The drawing under review shows one solid part. Ordinate dimensions are in mm from its lowest x, y, z. Coordinates: 2 decimals unless noted, no trailing zeros. Order: outer loops, then holes, each group sorted by start corner. A loop starts at its lowest first (then second) coordinate and runs counter-clockwise, first axis right, second up. Notation, with made-up numbers: (-33, 43) - (-11, 43) arc R35 ccw to (-11, 78) - close; hole circle Ø10 at (-13, 45.25). An arc over 180 degrees is marked (long way). Answer in a Markdown table with one row per item.
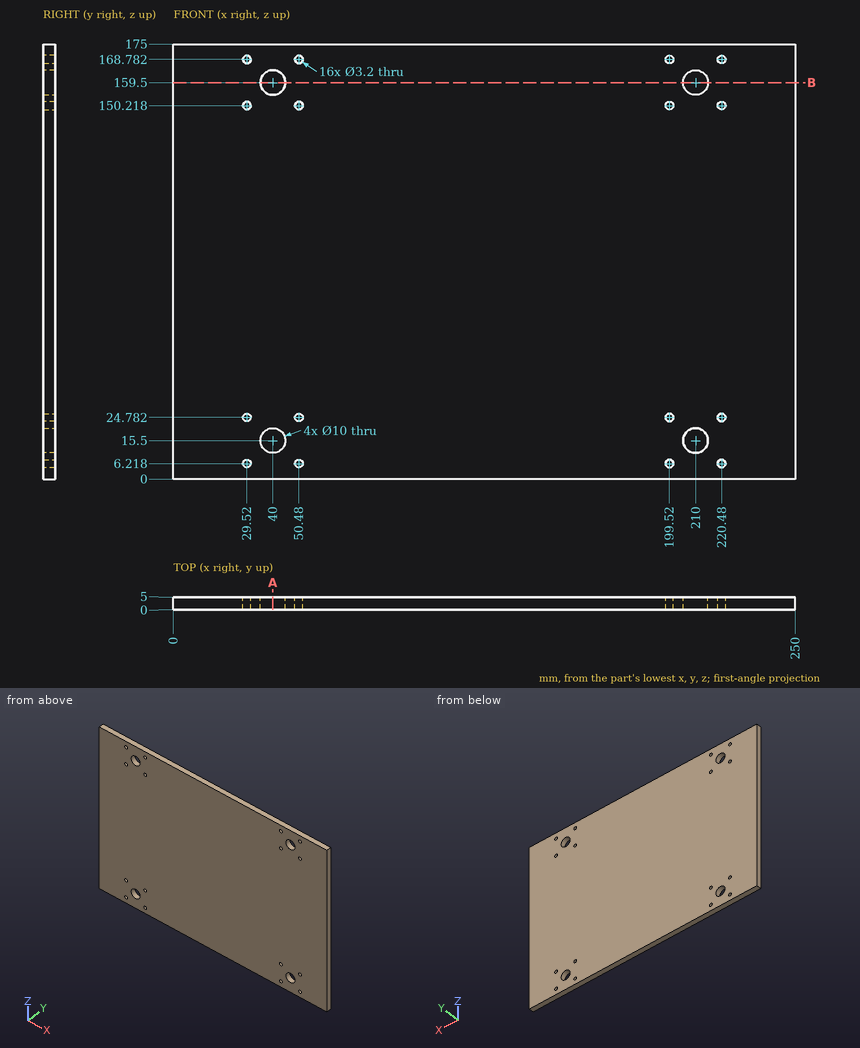
Item 1: We need section B-B, the plane z = 159.5. Write out the cut boundary in (x, y), then the cut area to 3 significant figures.
Check values:
| item | result |
|---|---|
| outline | (0, 0) - (35, 0) - (35, 5) - (0, 5) - close; (45, 0) - (205, 0) - (205, 5) - (45, 5) - close; (215, 0) - (250, 0) - (250, 5) - (215, 5) - close |
| area | 1,150 mm^2 |
Item 2: To check wall thickness, follow line 1 (X direction, y = 3.1, z = 159.5); line 2 (Z direction, x = 35.5, y = 2.8) (1 decimal); line 3 (X direction, y = 3.9, z = 162.5). State the ranges of each line that lie inside material, in increasing order. Write a range as from..to.
Check values:
| item | result |
|---|---|
| line 1 | 0..35, 45..205, 215..250 |
| line 2 | 0..13.3, 17.7..157.3, 161.7..175 |
| line 3 | 0..36, 44..206, 214..250 |
Item 3: We need section A-A, the plane x = 40. Write out the cut boundary in (y, z).
Check values:
| item | result |
|---|---|
| outline | (0, 0) - (5, 0) - (5, 10.5) - (0, 10.5) - close; (0, 20.5) - (5, 20.5) - (5, 154.5) - (0, 154.5) - close; (0, 164.5) - (5, 164.5) - (5, 175) - (0, 175) - close |
Item 4: Clearance check with a flat-ended pin moving along its axis: pin 1 Ø5 at (x, z) = (50.48, 150.22) entering from +Y. State where the tip first meets the part, or that it passes through.
Check values:
| item | result |
|---|---|
| pin 1 | y = 5 |
